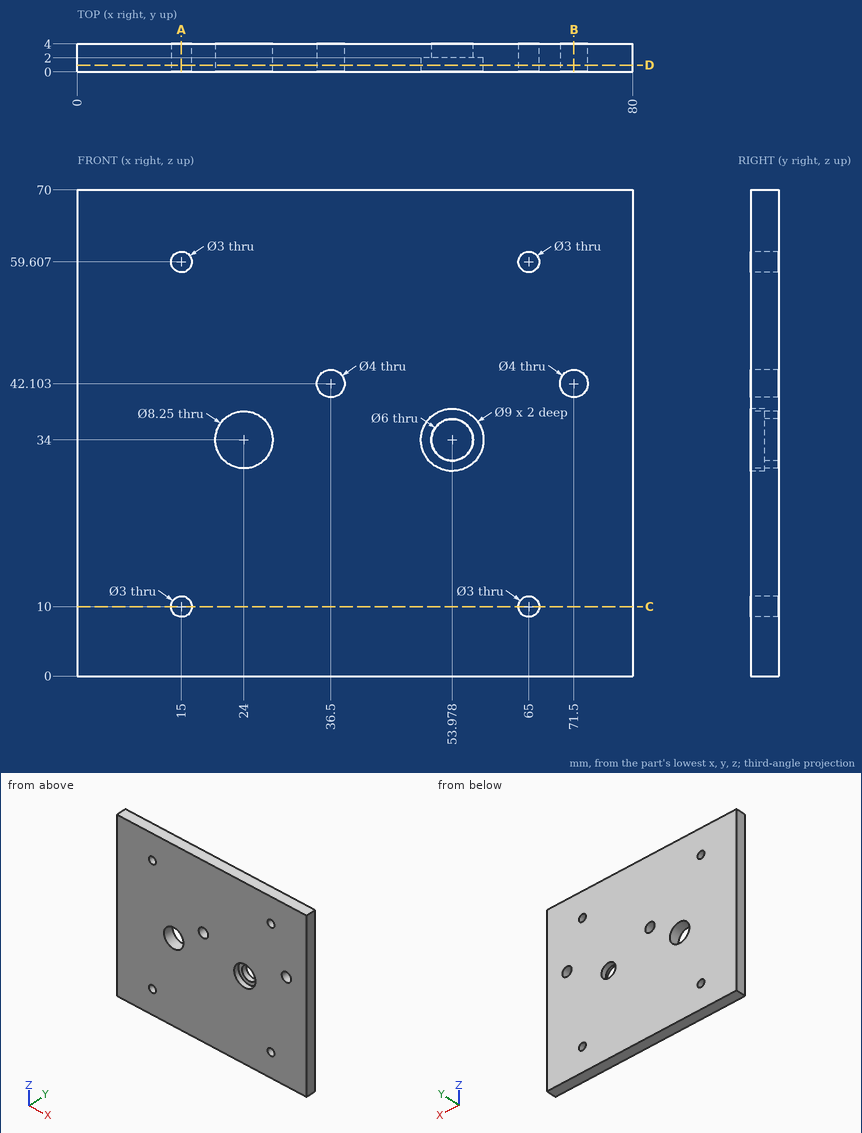
Here's the drawing with two shaded views (mm, measured from the low corner). I have some questions. Coordinates: 2 decimals unless noted, no trailing zeros. Loops run counter-clockwise (first coordinate to the right, second up) from the corner with the lowest first, then second, coordinate; pieces in that order, holes last. Notation, with made-up numbers: (29, 61) -> (78, 61) arc R23 cw to (78, 93) -> close; hole circle Ø9 at (68.5, 79.5). An arc over 180 degrees is marked (long way). Answer in a Markdown table with one row per item.
(1) If I drill on probe 1 along Z at (x, y) = (65, 1); probe 2 along X at (y, z) = (0.4, 32); probe 3 along Z at (x, y) = (71.5, 1.8), over which ranges is the centre line in solid material (lowest first)?
Results found:
| item | result |
|---|---|
| probe 1 | z = 0 to 8.5, 11.5 to 58.11, 61.11 to 70 |
| probe 2 | x = 0 to 20.39, 27.61 to 49.95, 58.01 to 80 |
| probe 3 | z = 0 to 40.1, 44.1 to 70 |
(2) Imagine slicing it at B-B (x = 71.5). List the corners of the cut face in (y, z) for me.
Results found:
| item | result |
|---|---|
| outline | (0, 0) -> (4, 0) -> (4, 40.1) -> (0, 40.1) -> close; (0, 44.1) -> (4, 44.1) -> (4, 70) -> (0, 70) -> close |
(3) Imagine slicing it at A-A (x = 15). List the corners of the cut face in (y, z) for me, plus the area to 3 significant figures.
Results found:
| item | result |
|---|---|
| outline | (0, 0) -> (4, 0) -> (4, 8.5) -> (0, 8.5) -> close; (0, 11.5) -> (4, 11.5) -> (4, 58.11) -> (0, 58.11) -> close; (0, 61.11) -> (4, 61.11) -> (4, 70) -> (0, 70) -> close |
| area | 256 mm^2 |
(4) Imagine slicing it at D-D (y = 0.95). Give the number of separate pieces and of enclosed holes in the cut face, plus the area to 3 significant figures.
Results found:
| item | result |
|---|---|
| separate pieces | 1 |
| enclosed holes | 8 |
| area | 5,430 mm^2 |
(5) Imagine slicing it at C-C (z = 10). List the corners of the cut face in (x, y) for me.
Results found:
| item | result |
|---|---|
| outline | (0, 0) -> (13.5, 0) -> (13.5, 4) -> (0, 4) -> close; (16.5, 0) -> (63.5, 0) -> (63.5, 4) -> (16.5, 4) -> close; (66.5, 0) -> (80, 0) -> (80, 4) -> (66.5, 4) -> close |
(6) Will this pin go through, and if not, where does the flat tip stop? pin 1 Ø4.5 at (x, z) = (53.5, 36) entering from -Y.
Results found:
| item | result |
|---|---|
| pin 1 | stops at y = 2 |
